Answer from the drawing. Dimensions are ordinates in mm from the lowest x, y and z of the part. Give positions to 0.01 mm unless a question says otherwise; leave off trailing zeros. Order: outer loops, then holes, each group sorted by start corner. A loop starts at its lowest first (then second) coordinate and runs counter-clockwise, first axis right, second up. Notation, with made-up numbers: (42, 59.5) - (69, 59.5) arc R30 cw to (69, 98.5) - close; hole circle Ø3 at (71, -28.75). An arc over 180 degrees is marked (long way). Use a Markdown table: item, result. Add a question column.
1) The mould has two halves that part along Y. Classify the marked faces 1, 2 and 3: released by +Y, released by -Y, zero draft, split by the parting line, or undercut.
2) Flat-ended cylindrical pins translate along their axes: pin 1 (5 mm diameter, centred on y = 21.5, z = 1, fed in from -X); pin 2 (5 mm diameter, centred on y = 25, z = 3, fed in from -X); pin 3 (5 mm diameter, centred on x = 37, z = 1.5, fed in from -Y). Find the tip coordinate at first contact, or state that the pin passes through.
3) Find section A-A, the plane x = 25.5. Determine the outline of the cut face in (y, z).
4) Find section C-C, the plane z = 4.25. Determine the outline of the cut face in (x, y) (3 decimals), plus the area to 3 significant figures.
5) Find section D-D, the plane x = 6. Determine the outline of the cut face in (y, z), plus the area to 3 significant figures.
6) Straight lines are drawn through the part: line 1 (Y direction, x = 25.5, z = 5.5); line 2 (Y direction, x = 26.5, z = 2.75); line 3 (X direction, y = 21.5, z = 4.5). For each, find the intervals that lie inside material, in ascending order.
7) Find section B-B, the plane y = 25.5. Determine the outline of the cut face in (x, z), plus the area to 3 significant figures.
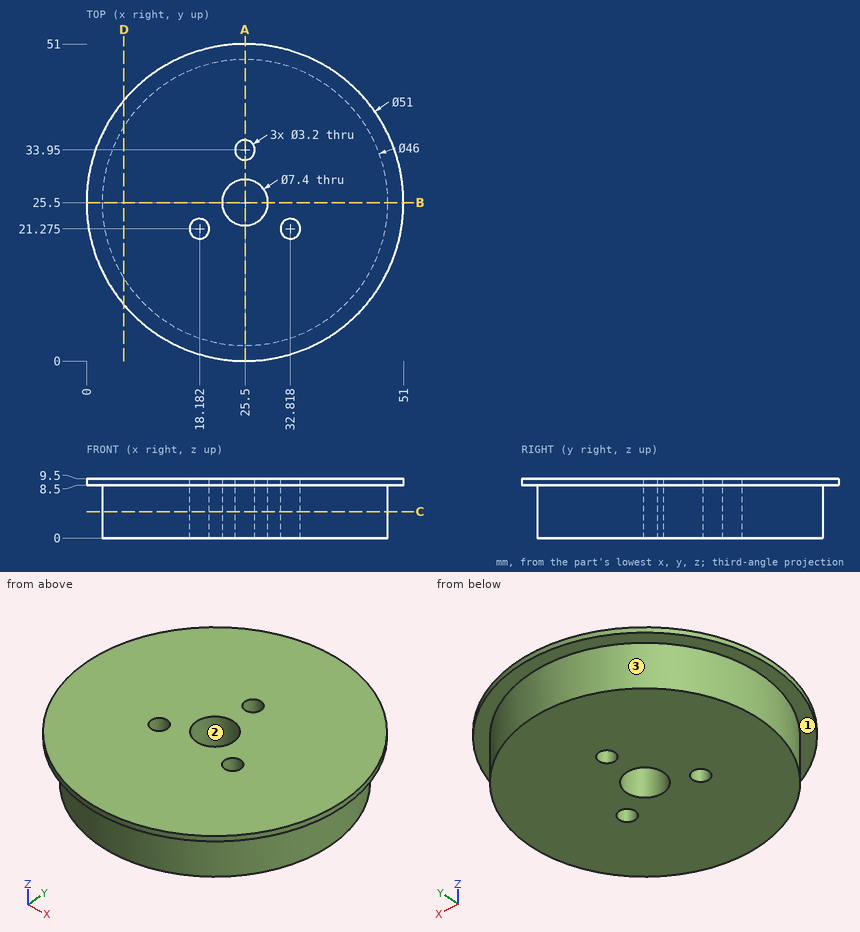
The answers:
| question | item | result |
|---|---|---|
| 1 | face 1 | zero draft |
| 1 | face 2 | undercut |
| 1 | face 3 | split by the parting line |
| 2 | pin 1 | x = 2.55 |
| 2 | pin 2 | x = 2.5 |
| 2 | pin 3 | y = 4.33 |
| 3 | outline | (0, 8.5) - (2.5, 8.5) - (2.5, 0) - (21.8, 0) - (21.8, 9.5) - (0, 9.5) - close; (29.2, 0) - (32.35, 0) - (32.35, 9.5) - (29.2, 9.5) - close; (35.55, 0) - (48.5, 0) - (48.5, 8.5) - (51, 8.5) - (51, 9.5) - (35.55, 9.5) - close |
| 4 | outline | circle Ø46 at (25.5, 25.5); hole circle Ø3.2 at (18.182, 21.275); hole circle Ø7.4 at (25.5, 25.5); hole circle Ø3.2 at (25.5, 33.95); hole circle Ø3.2 at (32.818, 21.275) |
| 4 | area | 1,590 mm2 |
| 5 | outline | (9.07, 8.5) - (13.3, 8.5) - (13.3, 0) - (37.7, 0) - (37.7, 8.5) - (41.93, 8.5) - (41.93, 9.5) - (9.07, 9.5) - close |
| 5 | area | 240 mm2 |
| 6 | line 1 | 2.5 to 21.8, 29.2 to 32.35, 35.55 to 48.5 |
| 6 | line 2 | 2.52 to 21.94, 29.06 to 32.7, 35.2 to 48.48 |
| 6 | line 3 | 2.85 to 16.6, 19.77 to 31.23, 34.4 to 48.15 |
| 7 | outline | (0, 8.5) - (2.5, 8.5) - (2.5, 0) - (21.8, 0) - (21.8, 9.5) - (0, 9.5) - close; (29.2, 0) - (48.5, 0) - (48.5, 8.5) - (51, 8.5) - (51, 9.5) - (29.2, 9.5) - close |
| 7 | area | 372 mm2 |
